Verification items for the finished model (mm, model axes). Face numbers are marked on the shaded views. A direction names the side the tool comes from. Coordinates: 2 decimals unless noted, no trailing zeros. Order: outer loops, then holes, each group sorted by start corner. A loop starts at its lowest first (then second) coordinate and runs counter-clockwise, first axis right, second up. Notation, with made-up numbers: M 67,69 L 115,69 A33 cw 115,106 Z; hole C 22,15.5 d11. An arc over 180 degrees is marked long. Write item = value, one per line.
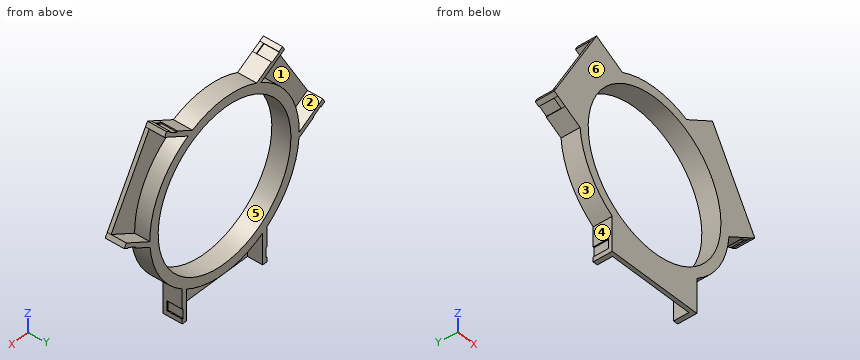
```python
from build123d import *

# Parameters (mm, degrees)
SKETCH1_R           = 40
BOSS_EXTRUDE1_DEPTH = 10
SKETCH2_R           = 40
BOSS_EXTRUDE2_DEPTH = 2


with BuildPart() as part:
    # Sketch1 → Boss-Extrude1 (new body)
    with BuildSketch(Plane(origin=(0, 0, 0), x_dir=(1, 0, 0), z_dir=(0, 1, 0))):
        with BuildLine():
            Line((-25.5, 37.077621283), (-25.5, 47.45))
            Line((-25.5, 47.45), (-25, 47.45))
            Line((-25, 47.45), (-25, 52.55))
            Line((-25, 52.55), (-25.5, 52.55))
            Line((-25.5, 52.55), (-25.5, 55.05))
            Line((-25.5, 55.05), (-23, 55.05))
            Line((-23, 55.05), (-23, 38.678159212))
            ThreePointArc((-23, 38.678159212), (0, 45), (23, 38.678159212))
            Line((23, 38.678159212), (23, 55.05))
            Line((23, 55.05), (25.5, 55.05))
            Line((25.5, 55.05), (25.5, 52.55))
            Line((25.5, 52.55), (25, 52.55))
            Line((25, 52.55), (25, 47.45))
            Line((25, 47.45), (25.5, 47.45))
            Line((25.5, 47.45), (25.5, 37.077621283))
            ThreePointArc((25.5, 37.077621283), (38.97114317, 22.5), (44.860161943, 3.544837155))
            Line((44.860161943, 3.544837155), (53.84290541, -1.641352203))
            Line((53.84290541, -1.641352203), (53.59290541, -2.074364905))
            Line((53.59290541, -2.074364905), (58.009634969, -4.624364905))
            Line((58.009634969, -4.624364905), (58.259634969, -4.191352203))
            Line((58.259634969, -4.191352203), (60.424698478, -5.441352203))
            Line((60.424698478, -5.441352203), (59.174698478, -7.606415713))
            Line((59.174698478, -7.606415713), (44.996268449, 0.579504681))
            ThreePointArc((44.996268449, 0.579504681), (38.97114317, -22.5), (21.996268449, -39.257663893))
            Line((21.996268449, -39.257663893), (36.174698478, -47.443584287))
            Line((36.174698478, -47.443584287), (34.924698478, -49.608647797))
            Line((34.924698478, -49.608647797), (32.759634969, -48.358647797))
            Line((32.759634969, -48.358647797), (33.009634969, -47.925635095))
            Line((33.009634969, -47.925635095), (28.59290541, -45.375635095))
            Line((28.59290541, -45.375635095), (28.34290541, -45.808647797))
            Line((28.34290541, -45.808647797), (19.360161943, -40.622458438))
            ThreePointArc((19.360161943, -40.622458438), (0, -45), (-19.360161943, -40.622458438))
            Line((-19.360161943, -40.622458438), (-28.34290541, -45.808647797))
            Line((-28.34290541, -45.808647797), (-28.59290541, -45.375635095))
            Line((-28.59290541, -45.375635095), (-33.009634969, -47.925635095))
            Line((-33.009634969, -47.925635095), (-32.759634969, -48.358647797))
            Line((-32.759634969, -48.358647797), (-34.924698478, -49.608647797))
            Line((-34.924698478, -49.608647797), (-36.174698478, -47.443584287))
            Line((-36.174698478, -47.443584287), (-21.996268449, -39.257663893))
            ThreePointArc((-21.996268449, -39.257663893), (-38.97114317, -22.5), (-44.996268449, 0.579504681))
            Line((-44.996268449, 0.579504681), (-59.174698478, -7.606415713))
            Line((-59.174698478, -7.606415713), (-60.424698478, -5.441352203))
            Line((-60.424698478, -5.441352203), (-58.259634969, -4.191352203))
            Line((-58.259634969, -4.191352203), (-58.009634969, -4.624364905))
            Line((-58.009634969, -4.624364905), (-53.59290541, -2.074364905))
            Line((-53.59290541, -2.074364905), (-53.84290541, -1.641352203))
            Line((-53.84290541, -1.641352203), (-44.860161943, 3.544837155))
            ThreePointArc((-44.860161943, 3.544837155), (-38.97114317, 22.5), (-25.5, 37.077621283))
        make_face()
        with Locations(Location((0, 0, 0), (0, 0, 270))):
            Circle(SKETCH1_R, mode=Mode.SUBTRACT)
    extrude(amount=BOSS_EXTRUDE1_DEPTH)

    # Sketch2 → Boss-Extrude2 (add)
    with BuildSketch(Plane.XZ):
        with BuildLine():
            Line((-60.424698478, 5.441352203), (-34.924698478, 49.608647797))
            Line((-34.924698478, 49.608647797), (-19.360161943, 40.622458438))
            ThreePointArc((-19.360161943, 40.622458438), (0, 45), (19.360161943, 40.622458438))
            Line((19.360161943, 40.622458438), (34.924698478, 49.608647797))
            Line((34.924698478, 49.608647797), (60.424698478, 5.441352203))
            Line((60.424698478, 5.441352203), (44.860161943, -3.544837155))
            ThreePointArc((44.860161943, -3.544837155), (38.97114317, -22.5), (25.5, -37.077621283))
            Line((25.5, -37.077621283), (25.5, -55.05))
            Line((25.5, -55.05), (-25.5, -55.05))
            Line((-25.5, -55.05), (-25.5, -37.077621283))
            ThreePointArc((-25.5, -37.077621283), (-38.97114317, -22.5), (-44.860161943, -3.544837155))
            Line((-44.860161943, -3.544837155), (-60.424698478, 5.441352203))
        make_face()
        with Locations(Location((0, 0, 0), (0, 0, 90))):
            Circle(SKETCH2_R, mode=Mode.SUBTRACT)
    extrude(amount=-BOSS_EXTRUDE2_DEPTH)


solid = part.part
```
Item 1: Sectioned sample at C-C, the plane x = 31. Enter the section's corners in (y, z).
Report:
outline = M 0,-32.62 L 10,-32.62 L 10,-25.28 L 0,-25.28 Z; M 0,25.28 L 10,25.28 L 10,32.62 L 2,32.62 L 2,44.46 L 10,44.46 L 10,46.77 L 2,46.77 L 2,47.34 L 0,47.34 Z
Item 2: Tool access check on the marked faces 1, 2 and 3. Record the directions out of +Z, -Z, +X, -X, +Y, -Y that give a thin tool (end or side, any length) a straight path to the whole face; none if there is none.
Report:
face_1 = +Y
face_2 = +Z, +Y
face_3 = -Z, -X, +Y, -Y
Item 3: Scan lines: L1, parallel to X at y = 3.5, z = 0; L2, parallel to Z at x = -26, y = 6.75; L3, parallel to Z at x = -16, y = 4.25. Record each from-to range of solid material in increasing order. Write a range as from..to.
Report:
L1 = -51..-46, -45..-40, 40..45, 46..51
L2 = -36.73..-30.4, 30.4..36.73, 41.57..44.46
L3 = -42.06..-36.66, 36.66..42.06
Item 4: Gauge pin test, flat ends, axial feed: pin 1 (4 mm diameter, centred on y = 8, z = -28, fed in from +X); pin 2 (4 mm diameter, centred on y = 6.5, z = -44.5, fed in from +X); pin 3 (4 mm diameter, centred on y = 5.5, z = -49.5, fed in from -X). Record the tip position at first contact, or that the pin passes through.
Report:
pin_1 = 36.73
pin_2 = 25.5
pin_3 = -25
Item 5: Sectioned sample at D-D, the plane z = -32. Enter the section's corners in (x, y), then the cut area to 3 significant figures.
Report:
outline = M -31.64,0 L -24,0 L -24,10 L -31.64,10 Z; M 24,0 L 31.64,0 L 31.64,10 L 24,10 Z
area = 153 mm^2
Item 6: Release check for a two-part mould opening along X. For the marked faces 4, 5 and 6 record: pulls with the +X half, pulls with the -X half, needs draft (parallel to the pull), parting line crosses it, or undercut.
Report:
face_4 = pulls with the -X half
face_5 = undercut
face_6 = needs draft
Item 7: Sectioned sample at A-A, the plane x = 0. Enter the section's corners in (y, z), then the cut area to 3 significant figures.
Report:
outline = M 0,-55.05 L 2,-55.05 L 2,-45 L 10,-45 L 10,-40 L 0,-40 Z; M 0,40 L 10,40 L 10,45 L 0,45 Z
area = 120 mm^2
Item 8: Sectioned sample at B-B, the plane z = -16. Enter the section's corners in (x, y).
Report:
outline = M -42.06,0 L -36.66,0 L -36.66,10 L -42.06,10 Z; M 36.66,0 L 42.06,0 L 42.06,10 L 36.66,10 Z
